For this review, take the finished solid that the model builds, in its own axes (mm). A direction names the side the tool comes from. Coordinates: 2 decimals unless noted, no trailing zeros. Loops run counter-clockwise (first coordinate to the right, second up) from the corner with the lowest first, then second, coordinate; pieces in that order, holes last.
1. Clearance check with flat-ended pins moving along their axes: P1, Ø1.5, axis at y = -2, z = 13, coming from the +X side; P2, Ø1, axis at y = -3, z = -16, coming from the -X side; P3, Ø3, axis at x = -2, y = -2.5, coming from the -Z side; P4, Ø1.9, axis at x = -3.57, z = 20.87, coming from the +Y side. State where each tip first meets the part, or that it passes through.
2. Mouldability with a two-part tool opening along X and no side actions: class faces 4 (the face through (0, -3, 14.327)), 5 (the face through (0, -6.35, 16)), 6 (the face through (-31.507, -3.131, 13.324)) as pulls with the +X half, pulls with the -X half, needs draft (parallel to the pull), parting line crosses it, or undercut.
3. Machinability: for faces 1 (the face through (-16.32, -3.13, -17.85)), 2 (the face through (0, 0, 16)), 3 (the face through (-13.592, -3.131, -37.614)), which of the approach directions +Z, -Z, +X, -X, +Y, -Y give a long, thin tool a straight path to every point of the face, cutting with its end or side? Answer none if there is none.
4. Take a section at C-C, the plane z = -19.5. State the section outline as (x, y) points.
5. To check wall thickness, follow probe 1 along X at (y, z) = (-2, 22); probe 2 along Z at (x, y) = (5.5, -0.5); probe 3 along X at (y, z) = (-1.75, 21). State the ranges of each line that lie inside material, in increasing order.
6. Take a section at B-B, the plane y = -2.5. State the section outline as (x, z) points (1 decimal).
7. Take a section at A-A, the plane z = 4. State the section outline as (x, y) points, then the cut area to 3 significant figures.
```python
from build123d import *

# Parameters (mm, degrees)
F1_DEPTH = 6.35
F3_D     = 3.175


with BuildPart() as f1:
    # F0 (on Front) → F1 (new body)
    with BuildSketch(Plane.XZ):
        Polygon((29.197415, 27.026769), (0, 27.026769), (0, 14.326769), (16.983994, 14.326769), (22.180271, 0), (10.29463, -36.19864), (16.983994, -39.069609), (33.752048, 0), align=None)
    extrude(amount=F1_DEPTH)

    # F3 (through all)
    with Locations(Plane.XZ.offset(6.35)):
        with Locations((3.570083, 20.865042)):
            Hole(F3_D / 2)

    # F4: F1 across plane


with BuildPart() as f1_1:
    add(f1.part)
    add(f1.part.mirror(Plane.YZ))


solid = f1_1.part
```
Results list:
1. P1: stops at x = 31.69
1. P2: stops at x = -27.1
1. P3: stops at z = 14.33
1. P4: passes through
2. face 4: undercut
2. face 5: needs draft
2. face 6: pulls with the -X half
3. face 1: +Y, -Y
3. face 2: +Z, -Z, +X, -X, +Y
3. face 3: -Z, +Y, -Y
4. outline: (-25.38, -6.35) - (-15.78, -6.35) - (-15.78, 0) - (-25.38, 0) - close; (15.78, -6.35) - (25.38, -6.35) - (25.38, 0) - (15.78, 0) - close
5. probe 1: x = -30.04 to -4.68, -2.46 to 2.46, 4.68 to 30.04
5. probe 2: z = 14.33 to 27.03
5. probe 3: x = -30.21 to -5.15, -1.99 to 1.99, 5.15 to 30.21
6. outline: (-33.8, 0) - (-17, -39.1) - (-10.3, -36.2) - (-22.2, 0) - (-17, 14.3) - (17, 14.3) - (22.2, 0) - (10.3, -36.2) - (17, -39.1) - (33.8, 0) - (29.2, 27) - (-29.2, 27) - close; hole circle Ø3.2 at (-3.6, 20.9); hole circle Ø3.2 at (3.6, 20.9)
7. outline: (-33.08, -6.35) - (-20.73, -6.35) - (-20.73, 0) - (-33.08, 0) - close; (20.73, -6.35) - (33.08, -6.35) - (33.08, 0) - (20.73, 0) - close
7. area: 157 mm2
